Geometry check sheet. Reference: the model listing, model coordinates, mm. A direction names the side the tool comes from. Give positions to 0.01 mm unless a question says otherwise; leave off trailing zeros. Order: outer loops, then holes, each group sorted by start corner. A loop starts at its lowest first (then second) coordinate and runs counter-clockwise, first axis right, second up. Notation, with made-up numbers: M 9,-18.5 L 47,-18.5 A12 cw 47,2.5 Z; hole C -38,-38.5 d4. An arc over 180 degrees is marked long. Answer as a JSON object with one key per item and string values. Group by question number.
from build123d import *

# Parameters (mm, degrees)
SZKIC1_W                                   = 60
SZKIC1_H                                   = 31
SZKIC1_R                                   = 12.5
DODANIE_WYCI_GNI_CIE1_DEPTH                = 5
SZKIC11_R                                  = 12.5
SZKIC11_R_2                                = 8.5
DODANIE_WYCI_GNI_CIE5_DEPTH                = 2
SZKIC7_W                                   = 2.5
SZKIC7_H                                   = 3
DODANIE_WYCI_GNI_CIE3_DEPTH                = 60
ZAOKR_GLENIE1_R                            = 3
WYTNIJ_WYCI_GNI_CIE1_DEPTH                 = 4
WYTNIJ_WYCI_GNI_CIE1_DEPTH_BACK            = 6
SZKIC3_R                                   = 21
SZKIC3_R_2                                 = 18
DODANIE_WYCI_GNI_CIE2_DEPTH                = 22
POG_BIENIE_STO_KOWE_POD_M2_5_RUB_Z_2_COUNT = 2
POG_BIENIE_STO_KOWE_POD_M2_5_RUB_Z_2_PITCH = 21.213203436
POG_BIENIE_STO_KOWE_POD_M2_5_RUB_Z_3_COUNT = 2
POG_BIENIE_STO_KOWE_POD_M2_5_RUB_Z_3_PITCH = 30
POG_BIENIE_STO_KOWE_POD_M2_5_RUB_Z_4_COUNT = 2
POG_BIENIE_STO_KOWE_POD_M2_5_RUB_Z_4_PITCH = 21.213203436
WYTNIJ_WYCI_GNI_CIE3_DEPTH                 = 4
DODANIE_WYCI_GNI_CIE4_DEPTH                = 1
WYTNIJ_WYCI_GNI_CIE2_DEPTH                 = 9


with BuildPart() as part:
    # Szkic1 → Dodanie-wyci_gni_cie1 (new body)
    with BuildSketch(Plane.XY):
        with Locations((-14, 0)):
            Rectangle(SZKIC1_W, SZKIC1_H)
        Circle(SZKIC1_R, mode=Mode.SUBTRACT)
    extrude(amount=DODANIE_WYCI_GNI_CIE1_DEPTH)

    # Szkic11 → Dodanie-wyci_gni_cie5 (add)
    with BuildSketch(Plane.XY.offset(5)):
        Circle(SZKIC11_R)
        Circle(SZKIC11_R_2, mode=Mode.SUBTRACT)
    extrude(amount=-DODANIE_WYCI_GNI_CIE5_DEPTH)

    # Szkic7 → Dodanie-wyci_gni_cie3 (add, through all)
    with BuildSketch(Plane.ZY.offset(44)):
        with Locations((1.25, 17)):
            Rectangle(SZKIC7_W, SZKIC7_H)
        with Locations((1.25, -17)):
            Rectangle(SZKIC7_W, SZKIC7_H)
        Polygon((5, -11.5), (5, -17.703597862), (8, -17.703597862), (8, -14.5), align=None)
    extrude(amount=-DODANIE_WYCI_GNI_CIE3_DEPTH)

    # Zaokr_glenie1
    zaokr_glenie1_edges = [part.edges().sort_by_distance(p)[0] for p in [
        (-14, -14.5, 8),
        (-14, -11.5, 5),
    ]]
    fillet(zaokr_glenie1_edges, radius=ZAOKR_GLENIE1_R)

    # Szkic2 → Wytnij-wyci_gni_cie1 (cut, two sides)
    with BuildSketch(Plane.XY.offset(5)) as wytnij_wyci_gni_cie1_sk:
        with BuildLine():
            Line((-25, -3.514225997), (-25, -20.5))
            Line((-25, -20.5), (-44, -20.5))
            Line((-44, -20.5), (-44, 35.715864495))
            ThreePointArc((-44, 35.715864495), (-30, 18.280268721), (-25, -3.514225997))
        make_face()
    extrude(amount=WYTNIJ_WYCI_GNI_CIE1_DEPTH, mode=Mode.SUBTRACT)
    extrude(wytnij_wyci_gni_cie1_sk.sketch, amount=-WYTNIJ_WYCI_GNI_CIE1_DEPTH_BACK, mode=Mode.SUBTRACT)

    # Szkic3 → Dodanie-wyci_gni_cie2 (add)
    with BuildSketch(Plane(origin=(0, 0, 0), x_dir=(-1, 0, 0), z_dir=(0, 0, -1))):
        Circle(SZKIC3_R)
        Circle(SZKIC3_R_2, mode=Mode.SUBTRACT)
    extrude(amount=DODANIE_WYCI_GNI_CIE2_DEPTH)

    # Szkic6 → Pog_bienie sto_kowe pod M2.5 _rub_ z _be (revolve, cut)
    with BuildSketch(Plane(origin=(-10.606601718, 10.606601718, 5), x_dir=(0, -1, 0), z_dir=(1, 0, 0))):
        Polygon((0, 0), (0, 27), (1.55, 27), (1.55, 1.2), (2.75, 0), align=None)
    pog_bienie_sto_kowe_pod_m2_5_rub_z_be = revolve(axis=Axis((-10.606601718, 10.606601718, 11.35), (0, 0, -1)), mode=Mode.SUBTRACT)

    # Pog_bienie sto_kowe pod M2.5 _rub_ z 2: Pog_bienie sto_kowe pod M2.5 _rub_ z _be ×2
    with Locations(*[(0, -i * POG_BIENIE_STO_KOWE_POD_M2_5_RUB_Z_2_PITCH, 0) for i in range(1, POG_BIENIE_STO_KOWE_POD_M2_5_RUB_Z_2_COUNT)]):
        add(pog_bienie_sto_kowe_pod_m2_5_rub_z_be, mode=Mode.SUBTRACT)

    # Pog_bienie sto_kowe pod M2.5 _rub_ z 3: Pog_bienie sto_kowe pod M2.5 _rub_ z _be ×2
    with Locations(*[Vector(0.707106781, -0.707106781, 0) * (i * POG_BIENIE_STO_KOWE_POD_M2_5_RUB_Z_3_PITCH) for i in range(1, POG_BIENIE_STO_KOWE_POD_M2_5_RUB_Z_3_COUNT)]):
        add(pog_bienie_sto_kowe_pod_m2_5_rub_z_be, mode=Mode.SUBTRACT)

    # Pog_bienie sto_kowe pod M2.5 _rub_ z 4: Pog_bienie sto_kowe pod M2.5 _rub_ z _be ×2
    with Locations(*[(i * POG_BIENIE_STO_KOWE_POD_M2_5_RUB_Z_4_PITCH, 0, 0) for i in range(1, POG_BIENIE_STO_KOWE_POD_M2_5_RUB_Z_4_COUNT)]):
        add(pog_bienie_sto_kowe_pod_m2_5_rub_z_be, mode=Mode.SUBTRACT)

    # Szkic15 → Wytnij-wyci_gni_cie3 (cut, through all)
    with BuildSketch(Plane.XY.offset(5)):
        with BuildLine():
            ThreePointArc((-13.334335162, -10.257359313), (-10.606601718, -13.356601718), (-7.878868274, -10.257359313))
            ThreePointArc((-7.878868274, -10.257359313), (-10.606601718, -7.856601718), (-13.334335162, -10.257359313))
        make_face()
        with BuildLine():
            ThreePointArc((7.878868274, -10.257359313), (10.606601718, -13.356601718), (13.334335162, -10.257359313))
            ThreePointArc((13.334335162, -10.257359313), (10.606601718, -7.856601718), (7.878868274, -10.257359313))
        make_face()
    extrude(amount=WYTNIJ_WYCI_GNI_CIE3_DEPTH, mode=Mode.SUBTRACT)

    # Szkic8 → Dodanie-wyci_gni_cie4 (add)
    with BuildSketch(Plane.XY):
        with BuildLine():
            Line((16, 13.601470509), (16, -13.601470509))
            ThreePointArc((16, -13.601470509), (21, 0), (16, 13.601470509))
        make_face()
    extrude(amount=DODANIE_WYCI_GNI_CIE4_DEPTH)

    # Szkic8_3 → Wytnij-wyci_gni_cie2 (cut, through all)
    with BuildSketch(Plane.XY):
        with BuildLine():
            ThreePointArc((9.937303457, 18.5), (13.19790989, 16.334478092), (16, 13.601470509))
            Line((16, 13.601470509), (16, 18.5))
            Line((16, 18.5), (9.937303457, 18.5))
        make_face()
        with BuildLine():
            Line((16, -18.5), (16, -13.601470509))
            ThreePointArc((16, -13.601470509), (13.19790989, -16.334478092), (9.937303457, -18.5))
            Line((9.937303457, -18.5), (16, -18.5))
        make_face()
    extrude(amount=WYTNIJ_WYCI_GNI_CIE2_DEPTH, mode=Mode.SUBTRACT)


solid = part.part
1. Release check for a two-part mould opening along Y. For faces 1 (the cylindrical face through (10.141, -12.085, 1.927)), 2 (the cylindrical face through (11.923, 3.755, 1.479)), 3 (the flat face through (-8, -18.5, 1)), 4 (the cylindrical face through (14.74, -11.39, 5.22)) record: released by +Y, released by -Y, zero draft, split by the parting line, or undercut.
2. Cross-section at D-D (y = 0). Record the cut outline in (x, z).
3. Cross-section at B-B (y = -16.5). Record the cut outline in (x, z), and give its area (3 significant figures).
4. Access from +Z, -Z, +X, -X, +Y, -Y to the whole of each face (thin tool, end or side, straight path). Record for faces 5 (the cylindrical face through (-9.66, -9.38, 1.93)), 6 (the flat face through (-3, -8.2, 3)), 7 (the flat face through (-8, 17, 2.5)), 8 (the flat face through (0, -19, 0)).
5. Thickness scan on line 1 along Y through (x, z) = (0, 1); line 2 along Z through (x, y) = (-9, -17.5); line 3 along Y through (x, z) = (0, 3.75). Record the ranges inside material, lowest first. Write a range as [from, to].
6. Depth check by flat-ended pin: pin 1 (9 mm diameter, centred on x = -10.61, y = -10.61, fed in from +Z); pin 2 (3 mm diameter, centred on x = 2, y = 19.5, fed in from +Z); pin 3 (1 mm diameter, centred on y = -16, z = -10.5, fed in from -X). Enter the tip coordinate at first touch or a pass-through.
7. Cross-section at C-C (z = -18). Record the cut outline in (x, y), and give its area (3 significant figures).
Report:
{
 "1": {"face 1": "undercut", "face 2": "undercut", "face 3": "released by -Y", "face 4": "released by +Y"},
 "2": {"outline": "M -25.12,0 L -21,0 L -21,-22 L -18,-22 L -18,0 L -12.5,0 L -12.5,3 L -8.5,3 L -8.5,5 L -25.12,5 Z; M 8.5,3 L 12.5,3 L 12.5,0 L 18,0 L 18,-22 L 21,-22 L 21,1 L 16,1 L 16,5 L 8.5,5 Z"},
 "3": {"outline": "M -25,0 L -12.99,0 L -12.99,-22 L -7.19,-22 L -7.19,0 L 7.19,0 L 7.19,-22 L 12.99,-22 L 12.99,2.5 L -25,2.5 Z; M -25,5 L 12.99,5 L 12.99,8 L -25,8 Z", "area": "464 mm2"},
 "4": {"face 5": "+Z, -Z", "face 6": "-Z", "face 7": "+Z, +X, -X, +Y", "face 8": "+Z, +X, -X, -Y"},
 "5": {"line 1": "y = [-18.5, -12.5], [12.5, 18.5]", "line 2": "z = [-22, 2.5], [5, 8]", "line 3": "y = [-15.5, -8.5], [8.5, 15.5]"},
 "6": {"pin 1": "stops at z = 7.93", "pin 2": "stops at z = 2.5", "pin 3": "stops at x = -14.17"},
 "7": {"outline": "C 0,0 d42; hole C 0,0 d36", "area": "368 mm2"}
}
